Here's the drawing with two shaded views (mm, measured from the low corner). I have some questions. Round coordinates to 2 decimals unless told otherwise and drop trailing zeros. Write each loop counter-clockwise with the first axis right and the second up, starting at its lowest first coordinate (ties: lowest second). Pieces come first, ordered by that corner, then holes. Notation, with made-up numbers: M -11.75,17 L 4.25,17 A24 cw 4.25,36 Z; hole C 35,54 d9. An arc over 180 degrees is marked long. Write item = value, one per line. Start each with the question number.
(1) I want a section at B-B (x = 172). List the corners of the cut face in (y, z) for me, and give its area (4 significant figures).
(2) Will these pins go through, and if not, where does the flat tip stop? pin 1 Ø3 at (x, z) = (298.5, 3) entering from -Y; pin 2 Ø6.5 at (y, z) = (111, 2) entering from +X.
(3) I need wall thicknesses on line 1 along X through (y, z) = (46.5, 4.75); line 2 along Y through (x, z) = (306, 5.5); line 3 along Z through (x, y) = (83, 165.5). Which ranges of each line are inside material? Lowest first, please.
(4) I want a section at A-A (y = 16). List the corners of the cut face in (x, z) for me, and give its area (3 significant figures).
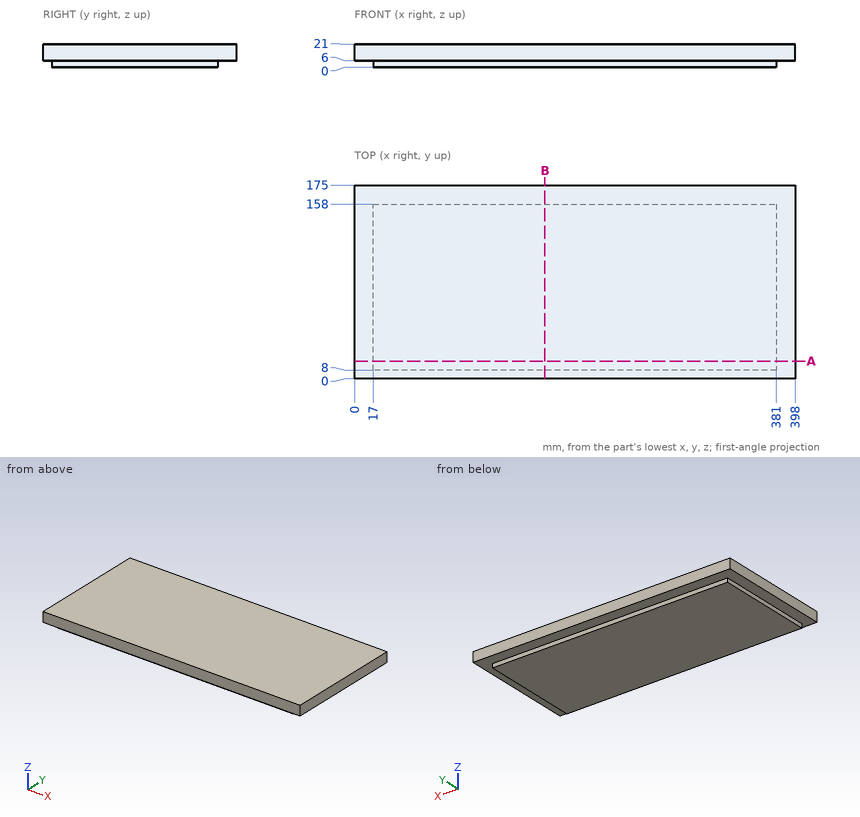
Returned:
q1.outline = M 0,6 L 8,6 L 8,0 L 158,0 L 158,6 L 175,6 L 175,21 L 0,21 Z
q1.area = 3,525 mm²
q2.pin_1 = 8
q2.pin_2 = 381
q3.line_1 = 17 to 381
q3.line_2 = 8 to 158
q3.line_3 = 6 to 21
q4.outline = M 0,6 L 17,6 L 17,0 L 381,0 L 381,6 L 398,6 L 398,21 L 0,21 Z
q4.area = 8,150 mm²
